Verification items for the finished model (mm, model axes). A direction names the side the tool comes from. Round coordinates to 2 decimals unless told otherwise and drop trailing zeros. Order: outer loops, then holes, each group sorted by start corner. A loop starts at its lowest first (then second) coordinate and runs counter-clockwise, first axis right, second up.
```python
from build123d import *

# Parameters (mm, degrees)
SKETCH1_W               = 20
SKETCH1_H               = 20
BOSS_EXTRUDE1_DEPTH     = 20
SKETCH2_R               = 3
CUT_EXTRUDE1_DEPTH      = 21
CHAMFER1_SIZE           = 0.5
CUT_EXTRUDE2_DEPTH      = 11
CUT_EXTRUDE2_DEPTH_BACK = 11
CUT_EXTRUDE3_DEPTH      = 11
CUT_EXTRUDE3_DEPTH_BACK = 11


with BuildPart() as part:
    # Sketch1 → Boss-Extrude1 (new body)
    with BuildSketch(Plane(origin=(0, 0, 0), x_dir=(1, 0, 0), z_dir=(0, 1, 0))):
        Rectangle(SKETCH1_W, SKETCH1_H)
    extrude(amount=BOSS_EXTRUDE1_DEPTH)

    # Sketch2 → Cut-Extrude1 (cut, through all)
    with BuildSketch(Plane.XY.offset(10)):
        with Locations((0, 10)):
            Circle(SKETCH2_R)
    extrude(amount=-CUT_EXTRUDE1_DEPTH, mode=Mode.SUBTRACT)

    # Chamfer1
    chamfer1_edges = [part.edges().sort_by_distance(p)[0] for p in [
        (-3, 10, -10),
        (-3, 10, 10),
    ]]
    chamfer(chamfer1_edges, length=CHAMFER1_SIZE)

    # Sketch3 → Cut-Extrude2 (cut, two sides)
    with BuildSketch(Plane.XY) as cut_extrude2_sk:
        Polygon((-3.5, 21), (-6, 18.5), (-8.5, 21), align=None)
        Polygon((2.5, 21), (0, 18.5), (-2.5, 21), align=None)
        Polygon((8.5, 21), (6, 18.5), (3.5, 21), align=None)
    extrude(amount=CUT_EXTRUDE2_DEPTH, mode=Mode.SUBTRACT)
    extrude(cut_extrude2_sk.sketch, amount=-CUT_EXTRUDE2_DEPTH_BACK, mode=Mode.SUBTRACT)

    # Sketch4 → Cut-Extrude3 (cut, two sides)
    with BuildSketch(Plane(origin=(0, 0, 0), x_dir=(0, 0, -1), z_dir=(1, 0, 0))) as cut_extrude3_sk:
        Polygon((-3.5, 21), (-6, 18.5), (-8.5, 21), align=None)
        Polygon((2.5, 21), (0, 18.5), (-2.5, 21), align=None)
        Polygon((8.5, 21), (6, 18.5), (3.5, 21), align=None)
    extrude(amount=CUT_EXTRUDE3_DEPTH, mode=Mode.SUBTRACT)
    extrude(cut_extrude3_sk.sketch, amount=-CUT_EXTRUDE3_DEPTH_BACK, mode=Mode.SUBTRACT)


solid = part.part
```
1) Tool access check on faces 1 (the flat face through (-0.6, 19.1, -3)), 2 (the flat face through (-3, 19.1, -0.6)), 3 (the flat face through (-9, 20, -3)). Record the directions out of +Z, -Z, +X, -X, +Y, -Y that give a thin tool (end or side, any length) a straight path to the whole face; none if there is none.
2) Sectioned sample at B-B on y = 10. Record the cut outline in (x, z), then the cut area to 4 significant figures.
3) Sectioned sample at A-A on z = -2.75. Record the cut outline in (x, y).
4) Go/stop test with flat-tipped pins: pin 1 Ø2 at (x, z) = (-6, 6) entering from +Y; pin 2 Ø3.5 at (x, y) = (0, 10) entering from +Z. Record where each tip stops, or that it passes through.
5) Scan lines: probe 1 along X at (y, z) = (8, 6.5); probe 2 along X at (y, z) = (9.5, 5.75); probe 3 along Y at (x, z) = (-1.5, 6.25). Record each from-to range of solid material in increasing order.
6) Sectioned sample at C-C on x = 8.25. Record the cut outline in (y, z).
Returned:
1. face 1: +Z, -Z, +Y
1. face 2: +X, -X, +Y
1. face 3: +Z, -Z, +X, -X, +Y
2. outline: (-10, -10) - (-3.5, -10) - (-3, -9.5) - (-3, 9.5) - (-3.5, 10) - (-10, 10) - close; (3, -9.5) - (3.5, -10) - (10, -10) - (10, 10) - (3.5, 10) - (3, 9.5) - close
2. area: 279.5 mm2
3. outline: (-10, 0) - (10, 0) - (10, 20) - (7.5, 20) - (6, 18.5) - (4.5, 20) - (1.5, 20) - (0, 18.5) - (-1.5, 20) - (-4.5, 20) - (-6, 18.5) - (-7.5, 20) - (-10, 20) - close; hole circle Ø6 at (0, 10)
4. pin 1: stops at y = 19.21
4. pin 2: passes through
5. probe 1: x = -10 to -2.24, 2.24 to 10
5. probe 2: x = -10 to -2.96, 2.96 to 10
5. probe 3: y = 0 to 7.4, 12.6 to 18.75
6. outline: (0, -10) - (20, -10) - (20, -7.5) - (18.5, -6) - (20, -4.5) - (20, -1.5) - (18.5, 0) - (20, 1.5) - (20, 4.5) - (18.5, 6) - (20, 7.5) - (20, 10) - (0, 10) - close
